Could you check a few things on this model? Use its own coordinates, in mm. Face numbers are marked on the shaded views. A direction names the side the tool comes from. Round coordinates to 2 decimals unless told otherwise and drop trailing zeros. Loops run counter-clockwise (first coordinate to the right, second up) from the corner with the lowest first, then second, coordinate; pieces in that order, holes last.
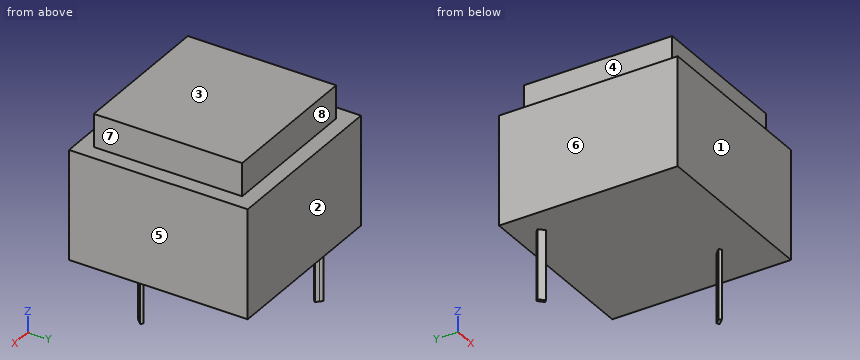
from build123d import *

# Parameters (mm, degrees)
F0_W     = 12.3952
F0_H     = 12.3952
F0_W_2   = 10.287
F0_H_2   = 10.287
F1_DEPTH = 7.5692
F2_DEPTH = 2.286
F4_DEPTH = 4.826


with BuildPart() as f1:
    # F0 (on Top) → F1 (new body)
    with BuildSketch(Plane.XY):
        with Locations((0.247709, -1.915304)):
            Rectangle(F0_W, F0_H)
        with Locations((0.247709, -1.915304)):
            Rectangle(F0_W_2, F0_H_2, mode=Mode.SUBTRACT)
        with Locations((0.247709, -1.915304)):
            Rectangle(F0_W_2, F0_H_2)
    extrude(amount=-F1_DEPTH)

    # F0 (on Top) → F2 (join)
    with BuildSketch(Plane.XY):
        with Locations((0.247709, -1.915304)):
            Rectangle(F0_W_2, F0_H_2)
    extrude(amount=F2_DEPTH)

    # F3 (on face) → F4 (join)
    with BuildSketch(Plane(origin=(0, 0, -7.5692), x_dir=(1, 0, 0), z_dir=(0, 0, -1))):
        Polygon((-4.40624, -2.594961), (-4.334398, -2.666803), (-4.171967, -2.504372), (-4.243809, -2.43253), align=None)
        Polygon((-4.171967, -2.504372), (-4.334398, -2.666803), (-4.262556, -2.738645), (-4.100125, -2.576214), align=None)
        Polygon((-4.171967, -2.504372), (-4.100125, -2.576214), (-3.903345, -2.379435), (-3.975187, -2.307593), align=None)
        Polygon((-4.047029, -2.23575), (-4.243809, -2.43253), (-4.171967, -2.504372), (-3.975187, -2.307593), align=None)
        Polygon((3.467957, 5.135552), (3.288352, 5.315157), (3.144668, 5.171473), (3.324273, 4.991868), align=None)
        Polygon((3.503878, 4.812263), (3.647562, 4.955947), (3.467957, 5.135552), (3.324273, 4.991868), align=None)
    extrude(amount=F4_DEPTH)


solid = f1.part
Item 1: If we section it at A-A, the plane z = -9.5: Please give me the cut outline in (x, y), then the cut area to 3 significant figures.
Results list:
outline: (-4.41, 2.59) - (-4.05, 2.24) - (-3.98, 2.31) - (-3.9, 2.38) - (-4.1, 2.58) - (-4.26, 2.74) - close; (3.14, -5.17) - (3.29, -5.32) - (3.65, -4.96) - (3.5, -4.81) - close
area: 0.206 mm2
Item 2: If we section it at D-D, the plane z = 1.25: Please give me the cut outline in (x, y), then the cut area to 3 significant figures.
Results list:
outline: (-4.9, -7.06) - (5.39, -7.06) - (5.39, 3.23) - (-4.9, 3.23) - close
area: 106 mm2
Item 3: We'd pull the mould along Y, two halves only. Please class the marked faces 1, 2 and 3: released by +Y, released by -Y, zero draft, split by the parting line, or undercut.
Results list:
face 1: released by -Y
face 2: released by +Y
face 3: zero draft
Item 4: Will these pins go through, and if not, where does the flat tip stop? pin 1 (3 mm diameter, centred on y = -6, z = -8, fed in from +X); pin 2 (1.1 mm diameter, centred on y = -1.5, z = 1, fed in from -X); pin 3 (3.5 mm diameter, centred on x = 2, y = 0, fed in from -Z); pin 4 (1.1 mm diameter, centred on y = -0.5, z = 1.5, fed in from +X).
Results list:
pin 1: stops at x = 6.45
pin 2: stops at x = -4.9
pin 3: stops at z = -7.57
pin 4: stops at x = 5.39
Item 5: If I drill on line 1 along Z through (x, y) = (-1.25, -6.5); line 2 along X through (y, z) = (-1.25, 1); line 3 along Z through (x, y) = (-1.25, 3.5), over which ranges is the centre line in solid material (lowest first)?
Results list:
line 1: z = -7.57 to 2.29
line 2: x = -4.9 to 5.39
line 3: z = -7.57 to 0
Item 6: For the marked faces 4, 5, 6, 7 and 8, which set-ups out of +Z, -Z, +X, -X, +Y, -Y let a thin tool reach every point of the face, with its end or its side?
Results list:
face 4: +Z, -X, +Y, -Y
face 5: +Z, -Z, +X, +Y, -Y
face 6: +Z, -Z, -X, +Y, -Y
face 7: +Z, +X, +Y, -Y
face 8: +Z, +X, -X, +Y
Item 7: If we section it at B-B, the plane y = 1: Please give me the cut outline in (x, z).
Results list:
outline: (-5.95, -7.57) - (6.45, -7.57) - (6.45, 0) - (5.39, 0) - (5.39, 2.29) - (-4.9, 2.29) - (-4.9, 0) - (-5.95, 0) - close
Item 8: If we section it at C-C, the plane x = -2.75: Please give me the cut outline in (y, z), then the cut area to 3 significant figures.
Results list:
outline: (-8.11, -7.57) - (4.28, -7.57) - (4.28, 0) - (3.23, 0) - (3.23, 2.29) - (-7.06, 2.29) - (-7.06, 0) - (-8.11, 0) - close
area: 117 mm2
